Geometry check sheet. Reference: the model listing, model coordinates, mm. A direction names the side the tool comes from. Give positions to 0.01 mm unless a question says otherwise; leave off trailing zeros. Order: outer loops, then holes, each group sorted by start corner. A loop starts at its lowest first (then second) coordinate and runs counter-clockwise, first axis right, second up. Notation, with made-up numbers: M 55.25,69.25 L 70.25,69.25 A21 ccw 70.25,104.25 Z; hole C 46.5,23 d11. An arc over 180 degrees is marked long. Put each result on its own line as item: value. Start each with the question number.
Q1. Go/stop test with flat-tipped pins: pin 1 (3.5 mm diameter, centred on x = 0, y = 13, fed in from -Z); pin 2 (1.8 mm diameter, centred on x = -8, z = 7.5, fed in from +Y); pin 3 (2 mm diameter, centred on y = 11.5, z = 3, fed in from +X); pin 4 (5.5 mm diameter, centred on y = 11, z = 0, fed in from -X). Record where each tip stops, or that it passes through.
Q2. Section check C-C on y = 6.5. Record the cut outline in (x, z), then the cut area to 3 significant figures.
Q3. Section check A-A on z = -7.5. Record the cut outline in (x, y), then the cut area to 3 significant figures.
Q4. Mould release check, pull along Z, two halves, no side actions. Record for faces 4 (the cylindrical face through (-9.464, 1.521, 7.175)), 5 (the cylindrical face through (7.1, 1.5, 6.3)), 6 (the cylindrical face through (-11.1, 1.52, 10.64)), 7 (the flat face through (0, 3, 5)): +Z half, -Z half, draft (parallel to the pull), parting line (faces both ways), or undercut.
Q5. Section check B-B on x = 3. Record the cut outline in (y, z).
Q6. Access from +Z, -Z, +X, -X, +Y, -Y to the whole of each face (thin tool, end or side, straight path). Record for faces 1 (the cylindrical face through (11.14, 1.52, 10.6)), 2 (the flat face through (0, 10, 3.5)), 3 (the flat face through (5, 9, 0)).
Q7. Section check D-D on z = 4.5. Record the cut outline in (x, y).
Q8. Material ranges on L1, parallel to X at y = 0.6, z = 7.5; L2, parallel to Y at x = 0, z = 0.5; L3, parallel to Z at x = -1, y = 16, recorded low to high.
```python
from build123d import *

# Parameters (mm, degrees)
SKETCH_1_W          = 24
SKETCH_1_H          = 23
EXTRUDE_1_DEPTH     = 3
SKETCH_2_W          = 10
SKETCH_2_H          = 7
EXTRUDE_2_DEPTH     = 15
SKETCH_3_R          = 1.5
CUT_EXTRUDE_2_DEPTH = 27.324893162
SKETCH_4_R          = 1.5
CUT_EXTRUDE_3_DEPTH = 23.388613177
FILLET_1_R          = 5
FILLET_2_R          = 3
FILLET_3_R          = 3


with BuildPart() as part:
    # 草图1 → 凸台-拉伸1 (new body)
    with BuildSketch(Plane(origin=(0, 0, 0), x_dir=(1, 0, 0), z_dir=(0, 1, 0))):
        Rectangle(SKETCH_1_W, SKETCH_1_H)
    extrude(amount=EXTRUDE_1_DEPTH)

    # 草图2 → 凸台-拉伸2 (add)
    with BuildSketch(Plane(origin=(0, 3, 0), x_dir=(1, 0, 0), z_dir=(0, 1, 0))):
        Rectangle(SKETCH_2_W, SKETCH_2_H)
    extrude(amount=EXTRUDE_2_DEPTH)

    # 草图3 → 切除-拉伸2 (cut, through all)
    with BuildSketch(Plane.XY.offset(3.5)):
        with Locations((0, 13)):
            Circle(SKETCH_3_R)
    extrude(amount=-CUT_EXTRUDE_2_DEPTH, mode=Mode.SUBTRACT)

    # 草图4 → 切除-拉伸3 (cut, through all)
    with BuildSketch(Plane(origin=(0, 3, 0), x_dir=(1, 0, 0), z_dir=(0, 1, 0))):
        with Locations(Location((-8, 7.5, 0), (0, 0, 270))):
            Circle(SKETCH_4_R)
        with Locations(Location((-8, -7.5, 0), (0, 0, 270))):
            Circle(SKETCH_4_R)
        with Locations(Location((8, -7.5, 0), (0, 0, 270))):
            Circle(SKETCH_4_R)
        with Locations(Location((8, 7.5, 0), (0, 0, 270))):
            Circle(SKETCH_4_R)
    extrude(amount=-CUT_EXTRUDE_3_DEPTH, mode=Mode.SUBTRACT)

    # 圆角1
    fillet_1_edges = [part.edges().sort_by_distance(p)[0] for p in [
        (-5, 18, 0),
        (5, 18, 0),
    ]]
    fillet(fillet_1_edges, radius=FILLET_1_R - 0.0001)  # a hair under: the kernel refuses the full size

    # 圆角2
    fillet_2_edges = [part.edges().sort_by_distance(p)[0] for p in [
        (5, 3, 0),
        (-5, 3, 0),
    ]]
    fillet(fillet_2_edges, radius=FILLET_2_R)

    # 圆角3
    fillet_3_edges = [part.edges().sort_by_distance(p)[0] for p in [
        (12, 1.5, 11.5),
        (-12, 1.5, 11.5),
        (-12, 1.5, -11.5),
        (12, 1.5, -11.5),
    ]]
    fillet(fillet_3_edges, radius=FILLET_3_R)


solid = part.part
```
Results found:
1. pin 1: stops at z = -3.5
1. pin 2: passes through
1. pin 3: stops at x = 5
1. pin 4: stops at x = -5
2. outline: M -5,-3.5 L 5,-3.5 L 5,3.5 L -5,3.5 Z
2. area: 70.0 mm^2
3. outline: M -12,0 L -9.5,0 L -9.5,3 L -12,3 Z; M -6.5,0 L 6.5,0 L 6.5,3 L -6.5,3 Z; M 9.5,0 L 12,0 L 12,3 L 9.5,3 Z
3. area: 54.0 mm^2
4. face 4: undercut
4. face 5: undercut
4. face 6: +Z half
4. face 7: draft
5. outline: M 0,-11.5 L 3,-11.5 L 3,-3.5 L 17,-3.5 L 17,3.5 L 3,3.5 L 3,11.5 L 0,11.5 Z
6. face 1: +Z, +X, +Y, -Y
6. face 2: +Z, +X, -X, +Y
6. face 3: +Z, -Z, +X, +Y
7. outline: M -12,0 L 12,0 L 12,3 L -12,3 Z
8. L1: x = -12 to -9.5, -6.5 to 6.5, 9.5 to 12
8. L2: y = 0 to 11.5, 14.5 to 18
8. L3: z = -3.5 to 3.5
